Could you check a few things on this drawing? It's one solid part, dimensions in mm from its lowest x, y, z. Round coordinates to 2 decimals unless told otherwise and drop trailing zeros. Write each loop counter-clockwise with the first axis right and the second up, starting at its lowest first coordinate (ties: lowest second). Pieces come first, ordered by that corner, then holes. Notation, with made-up numbers: M 77.25,16 L 125.25,16 A29 cw 125.25,55 Z; hole C 26.25,-19.5 d9. An arc over 180 degrees is marked long. One line per item, written item: value. Start each with the question number.
(1) I want a section at A-A on z = 5. Please give me the cut outline in (x, y).
(2) I want a section at C-C on x = 4.25. Please give me the cut outline in (y, z).
(3) Thinking about a two-plate mould opening in Y: for the marked faces 1, 2, 3 and 4, which applies, released by +Y, released by -Y, zero draft, split by the parting line, or undercut?
(4) If I drill on L1, parallel to Z at x = 7.5, y = 9.5; L2, parallel to Y at x = 3.75, z = 9.75; L3, parallel to Y at x = 1, z = 3, over which ranges is the centre line in solid material (lowest first)?
(5) I want a section at B-B on y = 5.5. Please give me the cut outline in (x, z).
(6) I want a section at D-D on x = 7.5. Please give me the cut outline in (y, z).
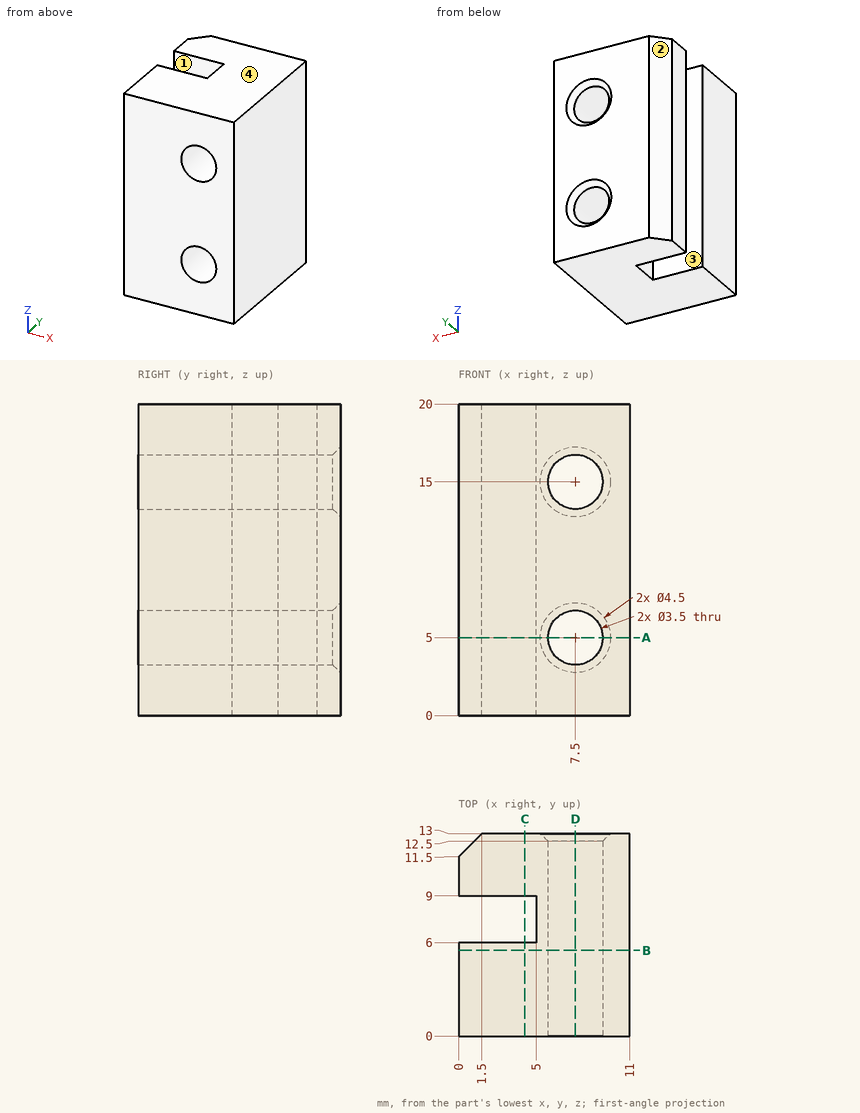
Found:
1. outline: M 0,0 L 5.75,0 L 5.75,12.5 L 5.25,13 L 1.5,13 L 0,11.5 L 0,9 L 5,9 L 5,6 L 0,6 Z; M 9.25,0 L 11,0 L 11,13 L 9.75,13 L 9.25,12.5 Z
2. outline: M 0,0 L 6,0 L 6,20 L 0,20 Z; M 9,0 L 13,0 L 13,20 L 9,20 Z
3. face 1: undercut
3. face 2: released by +Y
3. face 3: undercut
3. face 4: zero draft
4. L1: z = 0 to 3.25, 6.75 to 13.25, 16.75 to 20
4. L2: y = 0 to 6, 9 to 13
4. L3: y = 0 to 6, 9 to 12.5
5. outline: M 0,0 L 11,0 L 11,20 L 0,20 Z; hole C 7.5,5 d3.5; hole C 7.5,15 d3.5
6. outline: M 0,0 L 13,0 L 13,2.75 L 12.5,3.25 L 0,3.25 Z; M 0,6.75 L 12.5,6.75 L 13,7.25 L 13,12.75 L 12.5,13.25 L 0,13.25 Z; M 0,16.75 L 12.5,16.75 L 13,17.25 L 13,20 L 0,20 Z
